For this review, take the finished solid that the model builds, in its own axes (mm). Face numbers are marked on the shaded views. Round coordinates to 2 decimals unless told otherwise and drop trailing zeros. Order: outer loops, then holes, each group sorted by start corner. A loop starts at its lowest first (then second) coordinate and runs counter-clockwise, first axis right, second up. Notation, with made-up numbers: (23.25, 82) -> (53.25, 82) arc R20 cw to (53.25, 90) -> close; hole circle Ø8 at (57.5, 23). An arc over 180 degrees is marked (long way). Use a Markdown table: item, result. Add a question column.
1) Clearance check with flat-ended pins moving along their axes: P1, Ø4.5, axis at x = 0, y = 12.5, coming from the -Z side; P2, Ø3, axis at x = -18, y = 24, coming from the +Z side; P3, Ø6, axis at x = 11.5, z = 5.5, coming from the -Y side; P4, Ø10, axis at y = -25, z = 4.5, coming from the +X side. State where each tip first meets the part, or that it passes through.
2) Consider section C-C (x = 11). State the section outline as (y, z) points.
3) Consider section A-A (x = 0). State the section outline as (y, z) points.
4) Consider section B-B (z = 3). State the section outline as (x, y) points, plus the area to 3 significant figures.
5) Draft analysis for pull direction Y (two halves, no side actions). For the marked faces 1, 2 and 3, state which applies: pulls with the +Y half, pulls with the -Y half, needs draft (parallel to the pull), parting line crosses it, or undercut.
6) Wall thickness on line 1 along Y through (x, z) = (0, 2); line 2 along X through (y, z) = (-0.5, 6.25); line 3 along Z through (x, y) = (18, 6): over which ranges is each line inside the solid? List them lowest first. Write a range as [from, to].
```python
from build123d import *

# Parameters (mm, degrees)
CROQUIS1_R              = 32
CROQUIS1_R_2            = 5
SALIENTE_EXTRUIR1_DEPTH = 8
CROQUIS3_R              = 2.5
CORTAR_EXTRUIR1_DEPTH   = 10
CROQUIS4_R              = 4
SALIENTE_EXTRUIR2_DEPTH = 10


with BuildPart() as part:
    # Croquis1 → Saliente-Extruir1 (new body)
    with BuildSketch(Plane.XY):
        Circle(CROQUIS1_R)
        Circle(CROQUIS1_R_2, mode=Mode.SUBTRACT)
    extrude(amount=SALIENTE_EXTRUIR1_DEPTH)

    # Croquis3 → Cortar-Extruir1 (cut)
    with BuildSketch(Plane(origin=(0, 0, 0), x_dir=(-1, 0, 0), z_dir=(0, 0, -1))):
        with Locations((12.5, 0)):
            Circle(CROQUIS3_R)
        with Locations((0, -12.5)):
            Circle(CROQUIS3_R)
        with Locations((-12.5, 0)):
            Circle(CROQUIS3_R)
        with Locations((0, 12.5)):
            Circle(CROQUIS3_R)
    extrude(amount=-CORTAR_EXTRUIR1_DEPTH, mode=Mode.SUBTRACT)

    # Croquis4 → Saliente-Extruir2 (add)
    with BuildSketch(Plane.XY.offset(8)):
        with Locations((28, 0)):
            Circle(CROQUIS4_R)
    extrude(amount=SALIENTE_EXTRUIR2_DEPTH)


solid = part.part
```
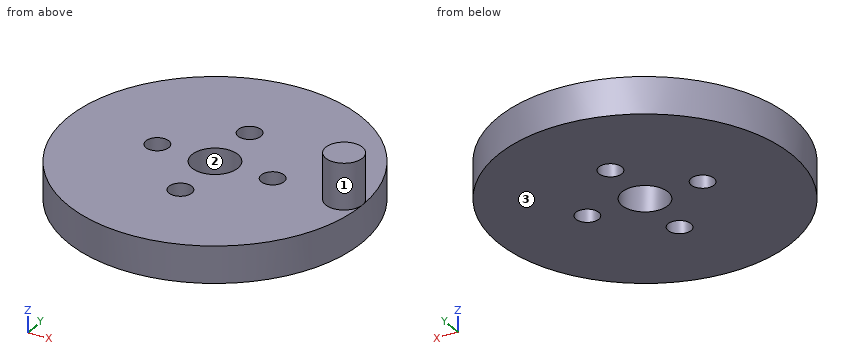
Results list:
| question | item | result |
|---|---|---|
| 1 | P1 | through |
| 1 | P2 | z = 8 |
| 1 | P3 | y = -30.85 |
| 1 | P4 | x = 24.98 |
| 2 | outline | (-30.05, 0) -> (-2, 0) -> (-2, 8) -> (-30.05, 8) -> close; (2, 0) -> (30.05, 0) -> (30.05, 8) -> (2, 8) -> close |
| 3 | outline | (-32, 0) -> (-15, 0) -> (-15, 8) -> (-32, 8) -> close; (-10, 0) -> (-5, 0) -> (-5, 8) -> (-10, 8) -> close; (5, 0) -> (10, 0) -> (10, 8) -> (5, 8) -> close; (15, 0) -> (32, 0) -> (32, 8) -> (15, 8) -> close |
| 4 | outline | circle Ø64 at (0, 0); hole circle Ø5 at (-12.5, 0); hole circle Ø10 at (0, 0); hole circle Ø5 at (0, -12.5); hole circle Ø5 at (0, 12.5); hole circle Ø5 at (12.5, 0) |
| 4 | area | 3,060 mm2 |
| 5 | face 1 | parting line crosses it |
| 5 | face 2 | undercut |
| 5 | face 3 | needs draft |
| 6 | line 1 | [-32, -15], [-10, -5], [5, 10], [15, 32] |
| 6 | line 2 | [-32, -14.95], [-10.05, -4.97], [4.97, 10.05], [14.95, 32] |
| 6 | line 3 | [0, 8] |
